from build123d import *

# Parameters (mm, degrees)
EXTRUDE_1_DEPTH     = 5
SKETCH_2_R          = 28
CUT_EXTRUDE_1_DEPTH = 91.840456458
SKETCH_3_W          = 19
SKETCH_3_H          = 30
CUT_EXTRUDE_2_DEPTH = 91.840456458
FILLET_2_R          = 4.5
SKETCH_4_W          = 19
SKETCH_4_H          = 30
CUT_EXTRUDE_3_DEPTH = 5
FILLET_3_R          = 4.5
SKETCH_6_R          = 2.5
CUT_EXTRUDE_5_DEPTH = 91.840456458
FILLET_4_R          = 6
SKETCH_7_R          = 2.5
CUT_EXTRUDE_6_DEPTH = 91.840456458
SKETCH_8_R          = 2
CUT_EXTRUDE_7_DEPTH = 91.840456458


with BuildPart() as part:
    # 草图1 → 凸台-拉伸1 (new body)
    with BuildSketch(Plane.XY):
        with BuildLine():
            Line((-26, 29.123470654), (54, 29.123470654))
            Line((54, 29.123470654), (54, -32.876529346))
            ThreePointArc((54, -32.876529346), (14, -72.876529346), (-26, -32.876529346))
            Line((-26, -32.876529346), (-26, 29.123470654))
        make_face()
    extrude(amount=EXTRUDE_1_DEPTH)

    # 草图2 → 切除-拉伸1 (cut, through all)
    with BuildSketch(Plane.XY.offset(5)):
        with Locations((14, -32.876529346)):
            Circle(SKETCH_2_R)
    extrude(amount=-CUT_EXTRUDE_1_DEPTH, mode=Mode.SUBTRACT)

    # 草图3 → 切除-拉伸2 (cut, through all)
    with BuildSketch(Plane.XY.offset(5)):
        with Locations((44.5, 14.123470654)):
            Rectangle(SKETCH_3_W, SKETCH_3_H)
    extrude(amount=-CUT_EXTRUDE_2_DEPTH, mode=Mode.SUBTRACT)

    # 圆角2
    fillet_2_edges = [part.edges().sort_by_distance(p)[0] for p in [
        (54, -0.876529346, 2.5),
        (35, -0.876529346, 2.5),
    ]]
    fillet(fillet_2_edges, radius=FILLET_2_R)

    # 草图4 → 切除-拉伸3 (cut)
    with BuildSketch(Plane.XY.offset(5)):
        with Locations((-16.5, 14.123470654)):
            Rectangle(SKETCH_4_W, SKETCH_4_H)
    extrude(amount=-CUT_EXTRUDE_3_DEPTH, mode=Mode.SUBTRACT)

    # 圆角3
    fillet_3_edges = [part.edges().sort_by_distance(p)[0] for p in [
        (-26, -0.876529346, 2.5),
        (-7, -0.876529346, 2.5),
    ]]
    fillet(fillet_3_edges, radius=FILLET_3_R)

    # 草图6 → 切除-拉伸5 (cut, through all)
    with BuildSketch(Plane.XY.offset(5)):
        with Locations((-20, -7.876529346)):
            Circle(SKETCH_6_R)
        with Locations((48, -7.876529346)):
            Circle(SKETCH_6_R)
    extrude(amount=-CUT_EXTRUDE_5_DEPTH, mode=Mode.SUBTRACT)

    # 圆角4
    fillet_4_edges = [part.edges().sort_by_distance(p)[0] for p in [
        (35, 29.123470654, 2.5),
        (-7, 29.123470654, 2.5),
    ]]
    fillet(fillet_4_edges, radius=FILLET_4_R)

    # 草图7 → 切除-拉伸6 (cut, through all)
    with BuildSketch(Plane.XY.offset(5)):
        with Locations((14, -66.876529346)):
            Circle(SKETCH_7_R)
        with Locations((-5.984698578, -60.383107155)):
            Circle(SKETCH_7_R)
        with Locations((-18.335921554, -43.383107155)):
            Circle(SKETCH_7_R)
        with Locations((46.335921554, -43.383107155)):
            Circle(SKETCH_7_R)
        with Locations((33.984698578, -60.383107155)):
            Circle(SKETCH_7_R)
    extrude(amount=-CUT_EXTRUDE_6_DEPTH, mode=Mode.SUBTRACT)

    # 草图8 → 切除-拉伸7 (cut, through all)
    with BuildSketch(Plane.XY.offset(5)):
        with Locations((-2, 6.623470654)):
            Circle(SKETCH_8_R)
        with Locations((-2, 21.623470654)):
            Circle(SKETCH_8_R)
        with Locations((30, 21.623470654)):
            Circle(SKETCH_8_R)
        with Locations((30, 6.623470654)):
            Circle(SKETCH_8_R)
    extrude(amount=-CUT_EXTRUDE_7_DEPTH, mode=Mode.SUBTRACT)


solid = part.part
For this review, take the finished solid that the model builds, in its own axes (mm). A direction names the side the tool comes from. Round coordinates to 2 decimals unless told otherwise and drop trailing zeros. Write each loop counter-clockwise with the first axis right and the second up, starting at its lowest first coordinate (ties: lowest second). Pieces come first, ordered by that corner, then holes. Notation, with made-up numbers: M 10,88.25 L 29,88.25 A21 cw 29,104.25 Z; hole C -9.5,20.5 d2. An arc over 180 degrees is marked long. Write item = value, one per line. Start each with the question number.
(1) The part is to be moulded in two halves that separate along X. For faces 3 (the face through (31.85, 20.86, 2.54)), 4 (the face through (44, -0.877, 3)), 5 (the face through (-2.43, 19.67, 2.54)), 6 (the face through (-24.647, -2.16, 2.465)), say which applies: +X half, -X half, draft (parallel to the pull), parting line (faces both ways), or undercut.
(2) We need section B-B (z = 1.65). Give the number of separate pieces and of enclosed holes in the cut face, then the cut area to 3 significant figures.
(3) We need section D-D (y = -54). Give the boundary of the cut face in (x, z), then the cut area to 3 significant figures.
(4) For faces 1 (the face through (35, 13, 3)), 2 (the face through (14, 29.123, 2)), list the 3-axis set-ups (+Z, -Z, +X, -X, +Y, -Y) from which the entire face can be reached by the end or side of a thin tool; tool diameter is ignored.
(5) We need section A-A (x = 14). Give the boundary of the cut face in (y, z), then the cut area to 3 significant figures.
(6) Clearance check with flat-ended pins moving along their axes: pin 1 Ø1 at (x, z) = (15.5, 2) entering from -Y; pin 2 Ø1.5 at (x, z) = (-18, 2) entering from +Y; pin 3 Ø3 at (x, y) = (33.98, -60.38) entering from -Z; pin 4 Ø3 at (x, z) = (26, 2.5) entering from -Y. State where each tip first meets the part, or that it passes through.
(7) We need section C-C (y = -42). Give the boundary of the cut face in (x, z), then the cut area to 3 significant figures.
(8) For line 1 along Y through (x, z) = (14, 1.05); line 2 along Y through (x, z) = (30, 2.9); line 3 along Y through (x, z) = (-18, 0.95), list the stretches that pass through material, from the lowest coordinate up.
Results found:
q1.face_3 = undercut
q1.face_4 = draft
q1.face_5 = undercut
q1.face_6 = -X half
q2.separate_pieces = 1
q2.enclosed_holes = 12
q2.area = 3,670 mm²
q3.outline = M -19.97,0 L -4.38,0 L -4.38,5 L -19.97,5 Z; M 32.38,0 L 47.97,0 L 47.97,5 L 32.38,5 Z
q3.area = 156 mm²
q4.face_1 = +Z, -Z, +X, +Y
q4.face_2 = +Z, -Z, +X, -X, +Y
q5.outline = M -72.88,0 L -69.38,0 L -69.38,5 L -72.88,5 Z; M -64.38,0 L -60.88,0 L -60.88,5 L -64.38,5 Z; M -4.88,0 L 29.12,0 L 29.12,5 L -4.88,5 Z
q5.area = 205 mm²
q6.pin_1 = -72.86
q6.pin_2 = -0.88
q6.pin_3 = through
q6.pin_4 = -71.47
q7.outline = M -24.95,0 L -20.42,0 L -20.42,5 L -24.95,5 Z; M -16.25,0 L -12.47,0 L -12.47,5 L -16.25,5 Z; M 40.47,0 L 44.25,0 L 44.25,5 L 40.47,5 Z; M 48.42,0 L 52.95,0 L 52.95,5 L 48.42,5 Z
q7.area = 83.1 mm²
q8.line_1 = -72.88 to -69.38, -64.38 to -60.88, -4.88 to 29.12
q8.line_2 = -69.54 to -55.85, -9.9 to 4.62, 8.62 to 19.62, 23.62 to 29.04
q8.line_3 = -56.88 to -45.86, -40.91 to -9.38, -6.38 to -0.88
